Could you check a few things on this drawing? It's one solid part, dimensions in mm from its lowest x, y, z. Give positions to 0.01 mm unless a question says otherwise; leave off trailing zeros. Order: outer loops, then holes, each group sorted by start corner. A loop starts at its lowest first (then second) coordinate and runs counter-clockwise, first axis right, second up.
Item 1: I want a section at D-D, the plane y = 7.5. Write out the boundary of the cut face in (x, z).
Item 2: I want a section at C-C, the plane z = 3.75. Write out the boundary of the cut face in (x, y) (1 decimal).
Item 3: If we mould it in two halves opening along Y, with no side actions, what happens to the marked faces 1, 2 and 3? For each: +Y half, -Y half, draft (parallel to the pull), parting line (faces both ways), or undercut.
Item 4: If I drill on line 1 along X through (y, z) = (4, 10) (1 decimal); line 2 along Y through (x, z) = (3.25, 12) (1 decimal); line 3 along X through (y, z) = (4.75, 3.5) (1 decimal), over which ranges is the centre line in solid material (lowest first)?
Item 5: I want a section at B-B, the plane y = 5.5. Write out the boundary of the cut face in (x, z) (1 decimal).
Item 6: I'm going to push a flat-ended pin straight in: pin 1 Ø3.5 at (x, y) = (4.13, 4.13) entering from +Z. Where does the tip first touch, or does it pass through?
Item 7: I want a section at A-A, the plane x = 3. Write out the boundary of the cut face in (y, z) (1 decimal).
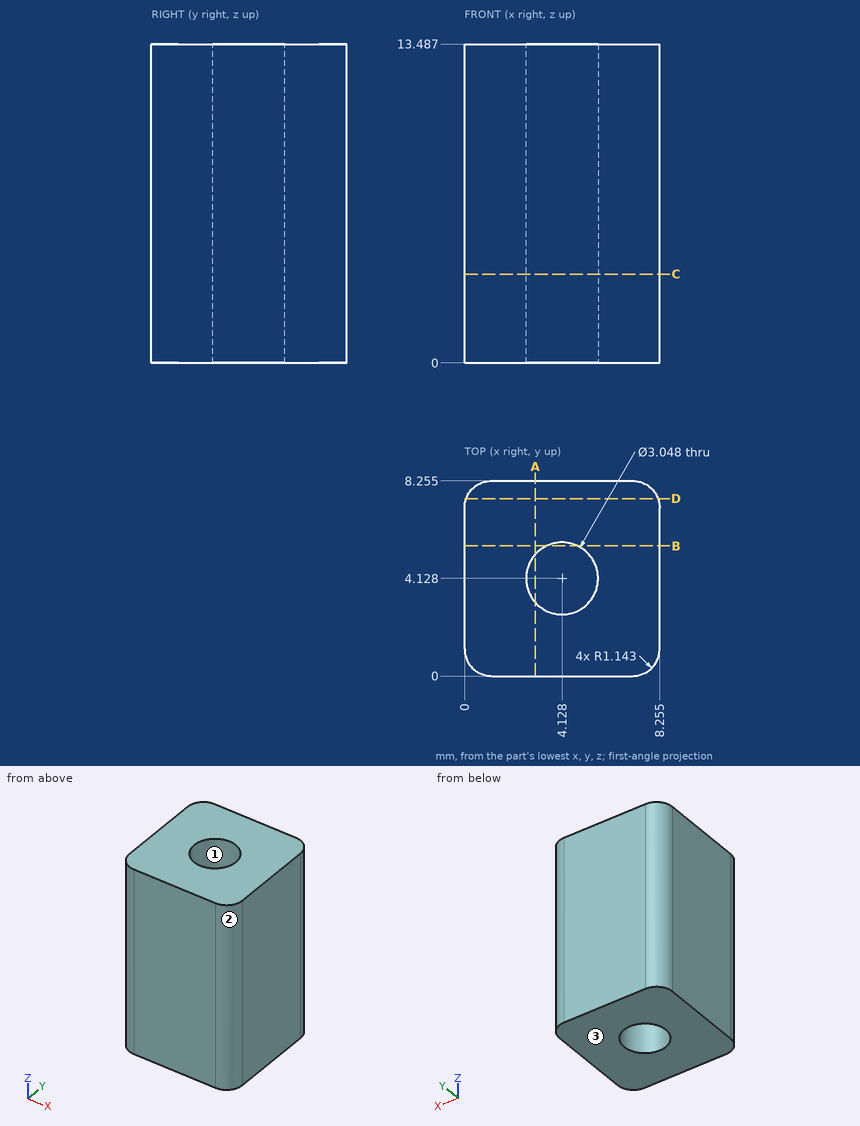
Results list:
1. outline: (0.07, 0) - (8.19, 0) - (8.19, 13.49) - (0.07, 13.49) - close
2. outline: (0, 1.1) arc R1.1 ccw to (1.1, 0) - (7.1, 0) arc R1.1 ccw to (8.3, 1.1) - (8.3, 7.1) arc R1.1 ccw to (7.1, 8.3) - (1.1, 8.3) arc R1.1 ccw to (0, 7.1) - close; hole circle Ø3 at (4.1, 4.1)
3. face 1: undercut
3. face 2: -Y half
3. face 3: draft
4. line 1: x = 0 to 2.6, 5.6 to 8.3
4. line 2: y = 0 to 2.9, 5.4 to 8.3
4. line 3: x = 0 to 2.7, 5.5 to 8.3
5. outline: (0, 0) - (3.5, 0) - (3.5, 13.5) - (0, 13.5) - close; (4.8, 0) - (8.3, 0) - (8.3, 13.5) - (4.8, 13.5) - close
6. pin 1: stops at z = 13.49
7. outline: (0, 0) - (3.1, 0) - (3.1, 13.5) - (0, 13.5) - close; (5.2, 0) - (8.3, 0) - (8.3, 13.5) - (5.2, 13.5) - close
